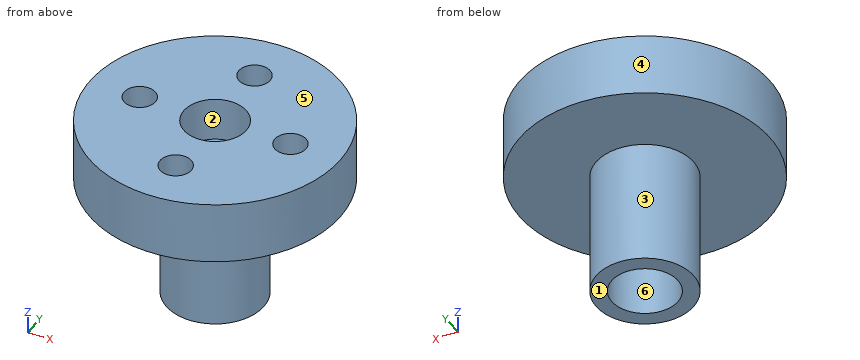
from build123d import *

# Parameters (mm, degrees)
SKETCH_1_R          = 3.9
SKETCH_1_R_2        = 2.65
EXTRUDE_1_DEPTH     = 10
SKETCH_3_R          = 10
EXTRUDE_2_DEPTH     = 5
SKETCH_5_R          = 1.25
CUT_EXTRUDE_1_DEPTH = 3
SKETCH_7_R          = 2.5
CUT_EXTRUDE_2_DEPTH = 3.5


with BuildPart() as part:
    # 草图1 → 凸台-拉伸1 (new body)
    with BuildSketch(Plane.XY):
        with Locations((0, 51.778341992)):
            Circle(SKETCH_1_R)
        with Locations((0, 51.778341992)):
            Circle(SKETCH_1_R_2, mode=Mode.SUBTRACT)
    extrude(amount=EXTRUDE_1_DEPTH)

    # 草图3 → 凸台-拉伸2 (add)
    with BuildSketch(Plane.XY.offset(10)):
        with Locations((0, 51.778341992)):
            Circle(SKETCH_3_R)
    extrude(amount=EXTRUDE_2_DEPTH)

    # 草图5 → 切除-拉伸1 (cut)
    with BuildSketch(Plane.XY.offset(15)):
        with Locations((6, 51.778341992)):
            Circle(SKETCH_5_R)
        with Locations((0, 57.778341992)):
            Circle(SKETCH_5_R)
        with Locations((0, 45.778341992)):
            Circle(SKETCH_5_R)
        with Locations((-6, 51.778341992)):
            Circle(SKETCH_5_R)
    extrude(amount=-CUT_EXTRUDE_1_DEPTH, mode=Mode.SUBTRACT)

    # 草图7 → 切除-拉伸2 (cut)
    with BuildSketch(Plane.XY.offset(15)):
        with Locations((0, 51.778341992)):
            Circle(SKETCH_7_R)
    extrude(amount=-CUT_EXTRUDE_2_DEPTH, mode=Mode.SUBTRACT)


solid = part.part
Check sheet for the modelled part. Datum: model origin and axes. Units: mm. Face numbers are marked on the shaded views. A direction names the side the tool comes from. Round coordinates to 2 decimals unless told otherwise and drop trailing zeros. Loops run counter-clockwise (first coordinate to the right, second up) from the corner with the lowest first, then second, coordinate; pieces in that order, holes last. Notation, with made-up numbers: (37.25, 41.5) - (92.25, 41.5) arc R25 cw to (92.25, 54.5) - close; hole circle Ø8 at (57.25, 45). An arc over 180 degrees is marked (long way). Answer as CSV lines item,"result". Start each with the question number.
Item 1: Section check D-D (z = 4.5). Record the boundary of the cut face in (x, y).
Item 2: Scan lines: line 1 (Y direction, x = -0.25, z = 14); line 2 (Z direction, x = 1.5, y = 44.75); line 3 (X direction, y = 52, z = 14). Record each from-to range of solid material in increasing order. Write a range as [from, to].
Item 3: Section check B-B (y = 53.75). Record the boundary of the cut face in (x, z).
Item 4: Section check C-C (z = 13.25). Record the boundary of the cut face in (x, y), and give its area (3 significant figures).
Item 5: Section check A-A (x = 0). Record the boundary of the cut face in (y, z).
Item 6: Release check for a two-part mould opening along X. For the marked faces 4, 5 and 6 record: +X half, -X half, draft (parallel to the pull), parting line (faces both ways), or undercut.
Item 7: Depth check by flat-ended pin: P1, Ø4, axis at x = -3, z = 7.5, coming from the -Y side; P2, Ø5.5, axis at x = 1, y = 51.5, coming from the +Z side; P3, Ø0.8, axis at x = 0, y = 46, coming from the +Z side; P4, Ø3, axis at x = 6, z = 10.5, coming from the +Y side. Enter the tip coordinate at first touch or a pass-through.
Item 8: Set-up check for the marked faces 1, 2 and 3: record each of +Z, -Z, +X, -X, +Y, -Y from which the full face is reachable in a straight line by a thin tool's end or side.
Report:
1,outline,"circle Ø7.8 at (0, 51.78); hole circle Ø5.3 at (0, 51.78)"
2,line 1,"y = [41.78, 44.55], [47, 49.29], [54.27, 56.55], [59, 61.78]"
2,line 2,"z = [10, 15]"
2,line 3,"x = [-10, -7.23], [-4.77, -2.49], [2.49, 4.77], [7.23, 10]"
3,outline,"(-9.8, 10) - (-3.36, 10) - (-3.36, 0) - (-1.77, 0) - (-1.77, 10) - (1.77, 10) - (1.77, 0) - (3.36, 0) - (3.36, 10) - (9.8, 10) - (9.8, 15) - (1.54, 15) - (1.54, 11.5) - (-1.54, 11.5) - (-1.54, 15) - (-9.8, 15) - close"
4,outline,"circle Ø20 at (0, 51.78); hole circle Ø2.5 at (-6, 51.78); hole circle Ø5 at (0, 51.78); hole circle Ø2.5 at (0, 45.78); hole circle Ø2.5 at (0, 57.78); hole circle Ø2.5 at (6, 51.78)"
4,area,"275 mm2"
5,outline,"(41.78, 10) - (47.88, 10) - (47.88, 0) - (49.13, 0) - (49.13, 10) - (54.43, 10) - (54.43, 0) - (55.68, 0) - (55.68, 10) - (61.78, 10) - (61.78, 15) - (59.03, 15) - (59.03, 12) - (56.53, 12) - (56.53, 15) - (54.28, 15) - (54.28, 11.5) - (49.28, 11.5) - (49.28, 15) - (47.03, 15) - (47.03, 12) - (44.53, 12) - (44.53, 15) - (41.78, 15) - close"
6,face 4,"parting line"
6,face 5,"draft"
6,face 6,"undercut"
7,P1,"stops at y = 48.01"
7,P2,"stops at z = 15"
7,P3,"stops at z = 12"
7,P4,"stops at y = 60.71"
8,face 1,"-Z, +X, -X, +Y, -Y"
8,face 2,"+Z"
8,face 3,"-Z"
